Source: three-view drawing plus pictorial views. Frame: mm from the lowest corner of the part. A direction names the side the tool comes from. Give positions to 0.01 mm unless a question says otherwise; leave off trailing zeros. Loops run counter-clockwise (first coordinate to the right, second up) from the corner with the lowest first, then second, coordinate; pieces in that order, holes last. Notation, with made-up numbers: (-31.5, 0) - (-26.5, 0) arc R15 ccw to (-26.5, 19) - close; hole circle Ø9 at (65.5, 77). An arc over 180 degrees is marked (long way). One line per item, written item: value.
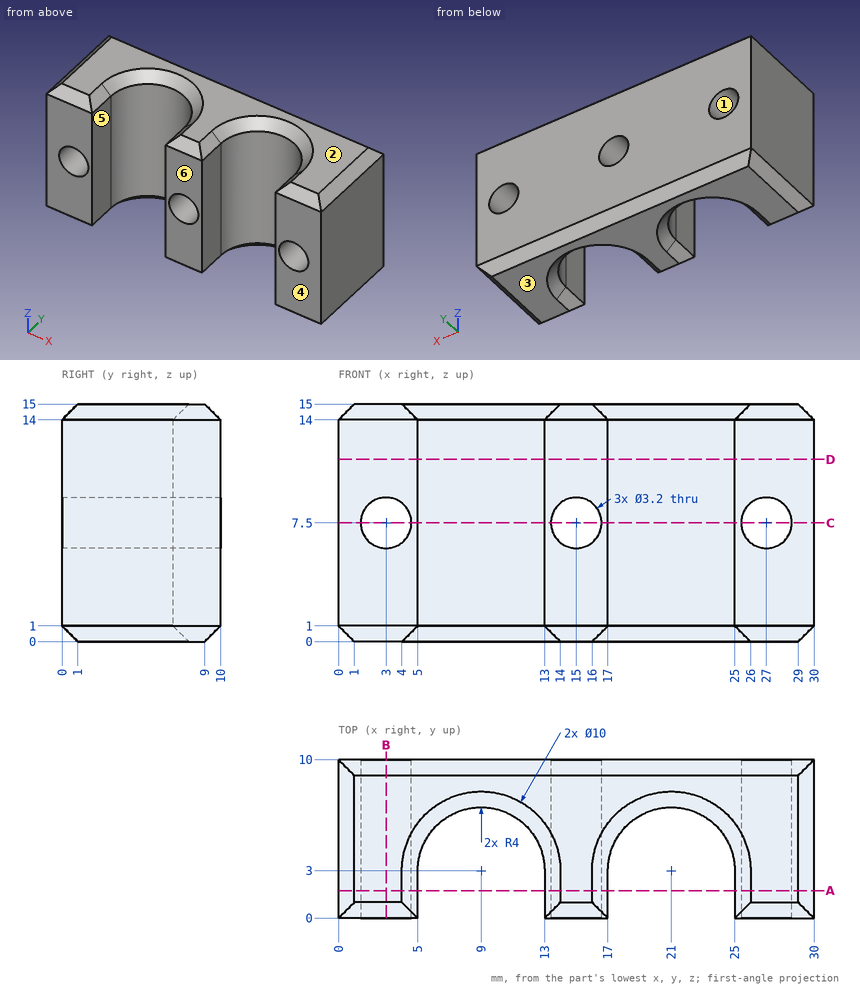
Item 1: Material intervals for L1, parallel to X at y = 1, z = 13.75; L2, parallel to Z at x = 27, y = 3.75; L3, parallel to X at y = 6.5, z = 11.25, sorted ascending.
Verdict:
L1: x = 0 to 5, 13 to 17, 25 to 30
L2: z = 0 to 5.9, 9.1 to 15
L3: x = 0 to 7.06, 10.94 to 19.06, 22.94 to 30
Item 2: Section D-D, the plane z = 11.5. Output: boundary loops of the cut face in (x, y).
Verdict:
outline: (0, 0) - (5, 0) - (5, 3) arc R4 cw to (13, 3) - (13, 0) - (17, 0) - (17, 3) arc R4 cw to (25, 3) - (25, 0) - (30, 0) - (30, 10) - (0, 10) - close
Item 3: Section A-A, the plane y = 1.75. Output: boundary loops of the cut face in (x, z), and give its area (3 significant figures).
Verdict:
outline: (0, 1) - (1, 0) - (4, 0) - (5, 1) - (5, 14) - (4, 15) - (1, 15) - (0, 14) - close; (13, 1) - (14, 0) - (16, 0) - (17, 1) - (17, 14) - (16, 15) - (14, 15) - (13, 14) - close; (25, 1) - (26, 0) - (29, 0) - (30, 1) - (30, 14) - (29, 15) - (26, 15) - (25, 14) - close; hole circle Ø3.2 at (3, 7.5); hole circle Ø3.2 at (15, 7.5); hole circle Ø3.2 at (27, 7.5)
area: 180 mm^2
Item 4: Draft query along Z for the marked faces 1, 2, 3 and 4. Return one class per face: pulls with the +Z half, pulls with the -Z half, needs draft (parallel to the pull), parting line crosses it, or undercut.
Verdict:
face 1: undercut
face 2: pulls with the +Z half
face 3: pulls with the -Z half
face 4: needs draft
Item 5: Section B-B, the plane x = 3. Output: boundary loops of the cut face in (y, z), and give its area (3 significant figures).
Verdict:
outline: (0, 1) - (1, 0) - (9, 0) - (10, 1) - (10, 5.9) - (0, 5.9) - close; (0, 9.1) - (10, 9.1) - (10, 14) - (9, 15) - (1, 15) - (0, 14) - close
area: 116 mm^2
Item 6: Section C-C, the plane z = 7.5. Output: boundary loops of the cut face in (x, y).
Verdict:
outline: (0, 0) - (1.4, 0) - (1.4, 10) - (0, 10) - close; (4.6, 0) - (5, 0) - (5, 3) arc R4 cw to (13, 3) - (13, 0) - (13.4, 0) - (13.4, 10) - (4.6, 10) - close; (16.6, 0) - (17, 0) - (17, 3) arc R4 cw to (25, 3) - (25, 0) - (25.4, 0) - (25.4, 10) - (16.6, 10) - close; (28.6, 0) - (30, 0) - (30, 10) - (28.6, 10) - close
Item 7: Pin query (flat end, axial travel): P1, Ø3, axis at y = 7, z = 11.5, coming from the -X side; P2, Ø1.5, axis at x = 10, y = 6.5, coming from the -Z side. Return the tip coordinate at first contact, or that it passes through.
Verdict:
P1: stops at x = 0
P2: stops at z = 0.61
Item 8: Access query for the marked faces 5 and 6. Directions: +Z, -Z, +X, -X, +Y, -Y. A direction counts if a zero-diameter tool reaches every point of the face in a straight line with its end or side. Return the directions, or none.
Verdict:
face 5: +Z, -Z, -Y
face 6: +Z, -Z, +X, -X, -Y
